Read the model definition and answer for the solid it produces. Units are mm, in the model's axes. A direction names the side the tool comes from. Give positions to 0.01 mm unless a question says otherwise; leave off trailing zeros. Loops run counter-clockwise (first coordinate to the right, second up) from the corner with the lowest first, then second, coordinate; pieces in that order, holes last. Notation, with made-up numbers: (84.5, 46) - (139.5, 46) arc R31 cw to (139.5, 73) - close; hole circle Ø8 at (-17.75, -36). An arc over 180 degrees is marked (long way). Write each question's results on one line, items separated by ' | '. Start each with the question number.
Q1. The part is cut by section B-B, the plane y = -17.5. Write down the section's boundary in (x, z), plus the area to 3 significant figures.
Q2. The part is cut by section C-C, the plane y = 0. Write down the section's boundary in (x, z).
Q3. The part is cut by section D-D, the plane x = -4. Write down the section's boundary in (y, z), plus the area to 3 significant figures.
Q4. The part is cut by section A-A, the plane z = 0.85. State how many separate pieces and enclosed holes the cut face has, plus the area to 3 significant figures.
Q5. Given pin 1 (1.5 mm diameter, centred on x = 14.5, y = -0.5, fed in from -Z); pin 2 (3 mm diameter, centred on x = 0, y = 8.5, fed in from +Z); pin 3 (1 mm diameter, centred on x = -15, z = 1, fed in from -Y), each flat-ended and moving along its own axis, determine where each tip first touches the part or whether it passes through.
Q6. For faces 1 (the cylindrical face through (12.932, 5.362, 2.24)), 2 (the cylindrical face through (-0.176, 7.161, 0.74)), determine the directions among +Z, -Z, +X, -X, +Y, -Y from which every point of the face is accessible in a straight line to the end or side of a thin tool.
Q7. Find the intervals of material crossed by line 1 (Y direction, x = 0, z = 0.9); line 2 (X direction, y = 8, z = 1.2); line 3 (X direction, y = -8.5, z = 1.75), in increasing order. Write a range as from..to.
Q8. Determine the mould class of faces 3 (the cylindrical face through (-14.093, 9.19, 1.479)), 4 (the flat face through (4, -4, 0)), 5 (the cylindrical face through (-2.799, -21.317, 1.479)) for opening direction Y: +Y half, -Y half, draft (parallel to the pull), parting line (faces both ways), or undercut.
Autodesk Inventor part; units mm, degrees
ref_plane "YZ Plane" through (0, 0, 0) normal (1, 0, 0) x (0, 1, 0)
ref_plane "XZ Plane" through (0, 0, 0) normal (0, 1, 0) x (-1, 0, 0)
ref_plane "XY Plane" through (0, 0, 0) normal (0, 0, 1) x (1, 0, 0)
sketch "スケッチ1" plane through (0, 0, 0) normal (0, 0, 1) x (1, 0, 0)
  circle A0 centre (0, 0) radius 21.5
  circle A1 centre (0, 0) radius 14
  line L0 (0, 21.5) -> (0, -21.5) construction
  circle A2 centre (0, 17.5) radius 1.15
  circle A3 centre (-15.1554, 8.75) radius 1.15
  circle A4 centre (-15.1554, -8.75) radius 1.15
  circle A5 centre (0, -17.5) radius 1.15
  circle A6 centre (15.1554, -8.75) radius 1.15
  circle A7 centre (15.1554, 8.75) radius 1.15
  circle A8 centre (0, 8.5) radius 1.35
  circle A9 centre (-8.5, 0) radius 1.35
  circle A10 centre (0, -8.5) radius 1.35
  circle A11 centre (8.5, 0) radius 1.35
  circle A12 centre (0, 0) radius 5.05
  dimension "d0" = 43
  dimension "d1" = 28
  dimension "d2" = 2.3
  dimension "d3" = 17.5
  dimension "d6" = 360
  dimension "d8" = 2.7
  dimension "d9" = 8.5
  dimension "d12" = 360
  dimension "d16" = 10.1
extrude "押し出し1" add sketch "スケッチ1" along normal blind 3 contours A0
extrude "押し出し2" add sketch "スケッチ1" along normal blind 1.5 contours A1
properties part number "Leg_joint_cross_bearing_frame" material "アルミニウム 2014-T4"
Check sheet entries:
1) outline: (-12.49, 0) - (-1.15, 0) - (-1.15, 3) - (-12.49, 3) - close; (1.15, 0) - (12.49, 0) - (12.49, 3) - (1.15, 3) - close | area: 68.0 mm^2
2) outline: (-21.5, 0) - (-9.85, 0) - (-9.85, 1.5) - (-14, 1.5) - (-14, 3) - (-21.5, 3) - close; (-7.15, 0) - (-5.05, 0) - (-5.05, 1.5) - (-7.15, 1.5) - close; (5.05, 0) - (7.15, 0) - (7.15, 1.5) - (5.05, 1.5) - close; (9.85, 0) - (21.5, 0) - (21.5, 3) - (14, 3) - (14, 1.5) - (9.85, 1.5) - close
3) outline: (-21.12, 0) - (-3.08, 0) - (-3.08, 1.5) - (-13.42, 1.5) - (-13.42, 3) - (-21.12, 3) - close; (3.08, 0) - (21.12, 0) - (21.12, 3) - (13.42, 3) - (13.42, 1.5) - (3.08, 1.5) - close | area: 77.3 mm^2
4) separate pieces: 1 | enclosed holes: 11 | area: 1,320 mm^2
5) pin 1: stops at z = 0 | pin 2: stops at z = 1.5 | pin 3: stops at y = -15.87
6) face 1: +Z | face 2: +Z, -Z
7) line 1: y = -21.5..-18.65, -16.35..-9.85, -7.15..-5.05, 5.05..7.15, 9.85..16.35, 18.65..21.5 | line 2: x = -19.96..-16.03, -14.28..-1.25, 1.25..14.28, 16.03..19.96 | line 3: x = -19.75..-16.28, -14.03..-11.12, 11.12..14.03, 16.28..19.75
8) face 3: undercut | face 4: draft | face 5: parting line
